Geometry check sheet. Reference: drawing and pictorial views, mm from the part's lowest x, y, z. A direction names the side the tool comes from. Coordinates: 2 decimals unless noted, no trailing zeros. Write each loop counter-clockwise with the first axis right and the second up, starting at its lowest first coordinate (ties: lowest second). Pieces come first, ordered by that corner, then holes. Notation, with made-up numbers: (-12, 70) -> (-8, 70) arc R20 cw to (-8, 81) -> close; hole circle Ø7 at (61.25, 87). An arc over 180 degrees is marked (long way). Answer in a Markdown table with one row per item.
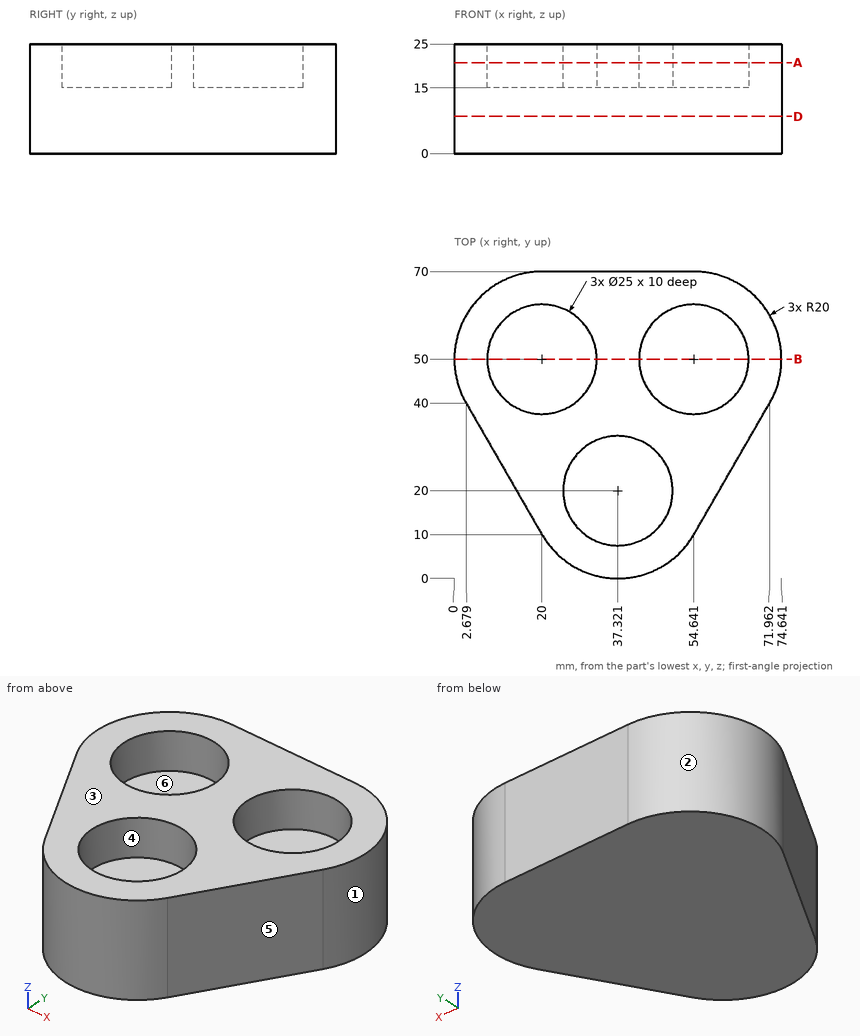
1. Tool access check on the marked faces 5 and 6. Record the directions out of +Z, -Z, +X, -X, +Y, -Y that give a thin tool (end or side, any length) a straight path to the whole face; none if there is none.
Geometry says:
| item | result |
|---|---|
| face 5 | +Z, -Z, +X, -Y |
| face 6 | +Z |
2. Section check B-B, the plane y = 50. Record the boundary of the cut face in (x, z).
Geometry says:
| item | result |
|---|---|
| outline | (0, 0) -> (74.64, 0) -> (74.64, 25) -> (67.14, 25) -> (67.14, 15) -> (42.14, 15) -> (42.14, 25) -> (32.5, 25) -> (32.5, 15) -> (7.5, 15) -> (7.5, 25) -> (0, 25) -> close |
3. Section check A-A, the plane z = 20.75. Record the boundary of the cut face in (x, y), plus the area to 3 significant figures.
Geometry says:
| item | result |
|---|---|
| outline | (2.68, 40) -> (20, 10) arc R20 ccw to (54.64, 10) -> (71.96, 40) arc R20 ccw to (54.64, 70) -> (20, 70) arc R20 ccw to start; hole circle Ø25 at (20, 50); hole circle Ø25 at (37.32, 20); hole circle Ø25 at (54.64, 50) |
| area | 2,380 mm^2 |
4. Depth check by flat-ended pin: P1, Ø4, axis at x = 46, y = 20, coming from the +Z side; P2, Ø8, axis at y = 47, z = 5, coming from the +X side; P3, Ø12, axis at y = 25.5, z = 18, coming from the -X side. Enter the tip coordinate at first touch or a pass-through.
Geometry says:
| item | result |
|---|---|
| P1 | z = 15 |
| P2 | x = 74.64 |
| P3 | x = 7.59 |
5. Mould release check, pull along X, two halves, no side actions. Record for the marked faces 1, 2, 3 and 4: released by +X, released by -X, zero draft, split by the parting line, or undercut.
Geometry says:
| item | result |
|---|---|
| face 1 | released by +X |
| face 2 | released by -X |
| face 3 | zero draft |
| face 4 | undercut |
6. Thickness scan on line 1 (Z direction, x = 48.5, y = 52.5); line 2 (Y direction, x = 41, z = 16.25) (1 decimal); line 3 (Y direction, x = 38, z = 9.75). Record the ranges inside material, lowest first. Write a range as from..to.
Geometry says:
| item | result |
|---|---|
| line 1 | 0..15 |
| line 2 | 0.3..8.1, 31.9..70 |
| line 3 | 0.01..70 |
7. Section check D-D, the plane z = 8.5. Record the boundary of the cut face in (x, y), plus the area to 3 significant figures.
Geometry says:
| item | result |
|---|---|
| outline | (2.68, 40) -> (20, 10) arc R20 ccw to (54.64, 10) -> (71.96, 40) arc R20 ccw to (54.64, 70) -> (20, 70) arc R20 ccw to start |
| area | 3,850 mm^2 |
